Geometry: see drawing. Coordinates: mm, zero at the bounding-box minimum. A direction names the side the tool comes from. Round coordinates to 2 decimals unless told otherwise and drop trailing zeros. Write each loop counter-clockwise with the first axis right and the second up, starting at its lowest first coordinate (ties: lowest second). Pieces come first, ordered by that corner, then holes. Notation, with made-up numbers: M 73,-28 L 106,-28 A19 cw 106,-8 Z; hole C 25.25,52.25 d8. An arc over 180 degrees is marked long. Use one line per item in the form item = value. Start each with the question number.
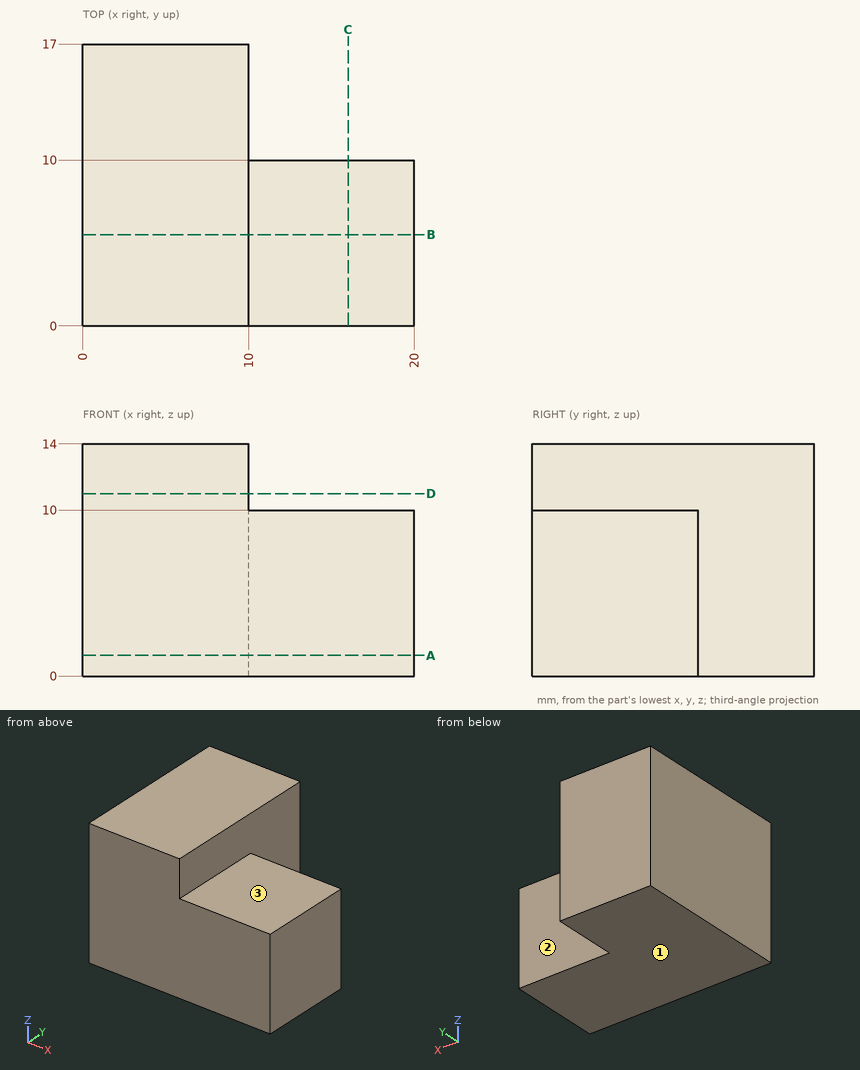
Item 1: Cut plane A-A (z = 1.25). Output: boundary loops of the cut face in (x, y), plus the area to 3 significant figures.
Item 2: Reachability of the marked faces 1, 2 and 3 from +Z, -Z, +X, -X, +Y, -Y: full face, straight path, thin tool, end or side. Return the list, or none.
Item 3: Cut plane D-D (z = 11). Output: boundary loops of the cut face in (x, y).
Item 4: Cut plane B-B (y = 5.5). Output: boundary loops of the cut face in (x, z), plus the area to 3 significant figures.
Item 5: Cut plane C-C (x = 16). Output: boundary loops of the cut face in (y, z), plus the area to 3 significant figures.
Item 6: Ray query, line 1 (Z direction, x = 14, y = 1.5). Return the intervals inside material, ascending. Write a range as from..to.
Item 7: First-contact query: pin 1 (5 mm diameter, centred on x = 13, y = 5.5, fed in from +Z); pin 2 (5 mm diameter, centred on x = 13.5, z = 2.5, fed in from +Y). Flat tips, straight axial feed; report the tip coordinate or a pass-through.
Final values:
q1.outline = M 0,0 L 20,0 L 20,10 L 10,10 L 10,17 L 0,17 Z
q1.area = 270 mm^2
q2.face_1 = -Z, +X, -X, +Y, -Y
q2.face_2 = +Z, -Z, +X, +Y
q2.face_3 = +Z, +X, +Y, -Y
q3.outline = M 0,0 L 10,0 L 10,17 L 0,17 Z
q4.outline = M 0,0 L 20,0 L 20,10 L 10,10 L 10,14 L 0,14 Z
q4.area = 240 mm^2
q5.outline = M 0,0 L 10,0 L 10,10 L 0,10 Z
q5.area = 100 mm^2
q6.line_1 = 0..10
q7.pin_1 = 10
q7.pin_2 = 10
